Answer from the drawing. Dimensions are ordinates in mm from the lowest x, y and z of the part. Coordinates: 2 decimals unless noted, no trailing zeros. Loops run counter-clockwise (first coordinate to the right, second up) from the corner with the lowest first, then second, coordinate; pieces in that order, holes last.
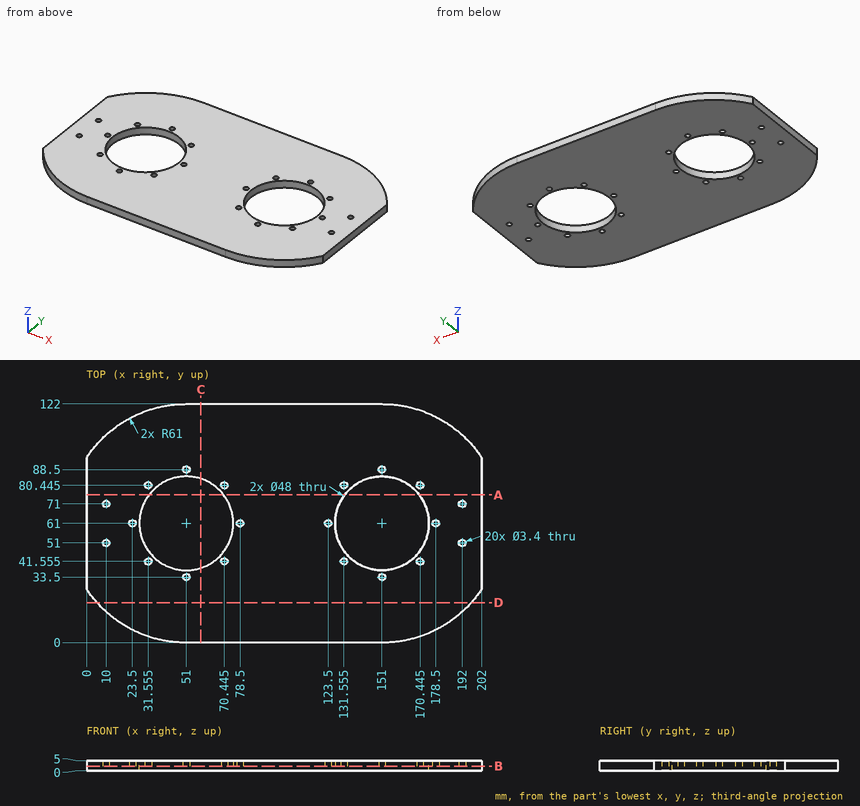
Item 1: A cutting plane is placed at A-A on y = 75.5. Determine the outline of the cut face in (x, z) (1 decimal).
Numbers:
outline: (0, 0) - (31.9, 0) - (31.9, 5) - (0, 5) - close; (70.1, 0) - (131.9, 0) - (131.9, 5) - (70.1, 5) - close; (170.1, 0) - (202, 0) - (202, 5) - (170.1, 5) - close
Item 2: Find the intervals of material crossed by line 1 along Y through (x, z) = (192, 2.55) (1 decimal); line 2 along Y through (x, z) = (31.5, 1.15) (1 decimal); line 3 along X through (y, z) = (88, 0.45) (1 decimal), in increasing order.
Numbers:
line 1: y = 15.8 to 49.3, 52.7 to 69.3, 72.7 to 106.2
line 2: y = 3.2 to 39.9, 43.3 to 47, 75 to 78.7, 82.1 to 118.8
line 3: x = 0 to 49.4, 52.6 to 149.4, 152.6 to 202
Item 3: Given pin 1 (4.5 mm diameter, centred on x = 10, y = 71, fed in from -Z); pin 2 (3 mm diameter, centred on y = 97, z = 2, fed in from +X); pin 3 (3 mm diameter, centred on y = 108, z = 3.5, fed in from -X); pin 4 (1.5 mm diameter, centred on x = 178.5, z = 1, fed in from +Y), each flat-ended and moving along its own axis, determine where each tip first touches the part or whether it passes through.
Numbers:
pin 1: stops at z = 0
pin 2: stops at x = 201.31
pin 3: stops at x = 10.37
pin 4: stops at y = 115.82
Item 4: A cutting plane is placed at D-D on y = 20.5. Determine the outline of the cut face in (x, z) (1 decimal), then the cut area to 3 significant figures.
Numbers:
outline: (5.4, 0) - (196.6, 0) - (196.6, 5) - (5.4, 5) - close
area: 956 mm2
Item 5: A cutting plane is placed at B-B on z = 2.2. Give the number of separate pieces and of enclosed holes in the cut face, then the cut area to 3 significant figures.
Numbers:
separate pieces: 1
enclosed holes: 22
area: 19,200 mm2
Item 6: A cutting plane is placed at C-C on x = 58.5. Determine the outline of the cut face in (y, z).
Numbers:
outline: (0, 0) - (38.2, 0) - (38.2, 5) - (0, 5) - close; (83.8, 0) - (122, 0) - (122, 5) - (83.8, 5) - close
